The listing builds one solid part. Answer for the finished solid, in the listing's coordinates (mm). Give positions to 0.01 mm unless a question says otherwise; leave off trailing zeros. Write each loop counter-clockwise with the first axis right and the second up, starting at its lowest first coordinate (ties: lowest second). Pieces come first, ordered by that corner, then holes. Notation, with made-up numbers: M 42.5,-29.75 L 46.5,-29.75 A5 ccw 46.5,-24.75 Z; hole C -13,8.5 d1. An arc over 180 degrees is marked long. Answer as a JSON object with one key per item and string values.
Autodesk Inventor part; units mm, degrees
ref_plane "YZ Plane" through (0, 0, 0) normal (1, 0, 0) x (0, 1, 0)
ref_plane "XZ Plane" through (0, 0, 0) normal (0, 1, 0) x (-1, 0, 0)
ref_plane "XY Plane" through (0, 0, 0) normal (0, 0, 1) x (1, 0, 0)
sketch "スケッチ1" plane through (0, 0, 0) normal (0, 1, 0) x (-1, 0, 0)
  circle A0 centre (0, 0) radius 31.75
  dimension "d0" = 63.5
extrude "押し出し1" add sketch "スケッチ1" along normal blind 5
sketch "スケッチ4" plane through (0, 5, 0) normal (0, 1, 0) x (1, 0, 0)
  circle A0 centre (0, 0) radius 17.5
  dimension "d9" = 35
extrude "押し出し4" cut sketch "スケッチ4" against normal through all
sketch "スケッチ6" plane through (0, 5, 0) normal (0, 1, 0) x (1, 0, 0)
  circle A0 centre (0, 0) radius 25 construction
  circle A1 centre (21.6506, 12.5) radius 2.15
  line L0 (0, 0) -> (21.6506, 12.5) construction
  line L1 (0, 0) -> (35.9214, 0) construction
  circle A2 centre (-21.6506, 12.5) radius 2.15
  circle A3 centre (0, -25) radius 2.15
  dimension "d19" = 50
  dimension "d20" = 4.3
  dimension "d21" = 30
  dimension "d24" = 360
extrude "押し出し6" cut sketch "スケッチ6" against normal through all
properties part number "B_probe_bearing_without_holes" material "PAEK 樹脂"
1. Consider line 1 along Z through (x, y) = (0, 2.15); line 2 along Z through (x, y) = (-26.5, 4.05); line 3 along X through (y, z) = (2.45, 25). Determine where each line is inside the solid, lowest interval first.
Verdict:
{"line 1": "z = -31.75 to -17.5, 17.5 to 22.85, 27.15 to 31.75", "line 2": "z = -17.49 to 17.49", "line 3": "x = -19.57 to -2.15, 2.15 to 19.57"}
2. A cutting plane is placed at A-A, the plane z = 0. Give the vertices of the cut face in (x, y), plus the area to 4 significant figures.
Verdict:
{"outline": "M -31.75,0 L -17.5,0 L -17.5,5 L -31.75,5 Z; M 17.5,0 L 31.75,0 L 31.75,5 L 17.5,5 Z", "area": "142.5 mm2"}
3. The mould has two halves that part along Z. Classify faces 1 (the cylindrical face through (-0.47, 2.54, 27.1)), 2 (the cylindrical face through (6.883, 2.465, 30.995)), 3 (the flat face through (-14, 5, -14)): released by +Z, released by -Z, zero draft, split by the parting line, or undercut.
Verdict:
{"face 1": "undercut", "face 2": "split by the parting line", "face 3": "zero draft"}
4. A cutting plane is placed at B-B, the plane x = 0. Give the vertices of the cut face in (y, z), plus the area to 3 significant figures.
Verdict:
{"outline": "M 0,-31.75 L 5,-31.75 L 5,-17.5 L 0,-17.5 Z; M 0,17.5 L 5,17.5 L 5,22.85 L 0,22.85 Z; M 0,27.15 L 5,27.15 L 5,31.75 L 0,31.75 Z", "area": "121 mm2"}
5. A cutting plane is placed at C-C, the plane y = 2.8. Give the vertices of the cut face in (x, z), plus the area to 3 significant figures.
Verdict:
{"outline": "C 0,0 d63.5; hole C -21.65,-12.5 d4.3; hole C 0,0 d35; hole C 0,25 d4.3; hole C 21.65,-12.5 d4.3", "area": "2,160 mm2"}
6. A cutting plane is placed at D-D, the plane z = -12.5. Give the vertices of the cut face in (x, y).
Verdict:
{"outline": "M -29.19,0 L -23.8,0 L -23.8,5 L -29.19,5 Z; M -19.5,0 L -12.25,0 L -12.25,5 L -19.5,5 Z; M 12.25,0 L 19.5,0 L 19.5,5 L 12.25,5 Z; M 23.8,0 L 29.19,0 L 29.19,5 L 23.8,5 Z"}
7. Flat-ended cylindrical pins translate along their axes: pin 1 (1 mm diameter, centred on y = 2.5, z = -3, fed in from -X); pin 2 (1 mm diameter, centred on x = -2, y = 4.5, fed in from -Z); pin 3 (1 mm diameter, centred on y = 3, z = 2, fed in from +X). Find the tip coordinate at first contact, or state that the pin passes through.
Verdict:
{"pin 1": "stops at x = -31.65", "pin 2": "stops at z = -31.71", "pin 3": "stops at x = 31.71"}
